For this review, take the finished solid that the model builds, in its own axes (mm). A direction names the side the tool comes from. Give positions to 0.01 mm unless a question says otherwise; leave off trailing zeros. Order: outer loops, then holes, each group sorted by start corner. A loop starts at its lowest first (then second) coordinate and runs counter-clockwise, first axis right, second up.
from build123d import *

# Parameters (mm, degrees)
F1_DEPTH = 25
F2_R     = 2
F4_DEPTH = 25


with BuildPart() as f1:
    # F0 (on Front) → F1 (new body)
    with BuildSketch(Plane.XZ):
        Polygon((3, 0), (0, 0), (-3, 0), (-3, -1), (-5, -3), (5, -3), (3, -1), align=None)
        Polygon((-3, 0), (0, 0), (3, 0), (3, 1), (-3, 1), align=None)
    extrude(amount=F1_DEPTH)

    # F2
    f2_edges = [f1.edges().sort_by_distance(p)[0] for p in [
        (-3, -25, 0),
        (-4, -25, -2),
        (4, -25, -2),
        (3, -25, 0),
        (-4, 0, -2),
        (3, 0, 0),
        (4, 0, -2),
        (-3, 0, 0),
    ]]
    fillet(f2_edges, radius=F2_R)

    # F3 (on face) → F4 (cut)
    with BuildSketch(Plane.XY.offset(1)):
        Polygon((-3, -12.972297), (-3, -12.5), (-3, -12.29), (-7.69, -12.29), (-7.69, -19.71), (-6.344625, -19.71), align=None)
        Polygon((-7.48, -12.5), (-3, -12.5), (-6.47483, -19.5), (-7.48, -19.5), align=None, mode=Mode.SUBTRACT)
        Polygon((-6.47483, -19.5), (-3, -12.5), (-7.48, -12.5), (-7.48, -19.5), align=None)
    extrude(amount=-F4_DEPTH, mode=Mode.SUBTRACT)


solid = f1.part
1) Tool access review of faces 4 (the face through (-2.43, -0.6, -0.12)), 5 (the face through (-3.5, -12.29, -2.4)), 6 (the face through (2.43, -24.4, -0.08)), 7 (the face through (2.43, -0.6, -0.08)), 8 (the face through (3, -12, 0)): name each direction out of +Z, -Z, +X, -X, +Y, -Y from which nothing blocks a thin tool from reaching the whole face with its end or side.
Answer sheet:
face 4: +Z, -X, +Y
face 5: +Z, -Z, -X
face 6: +Z, +X, -Y
face 7: +Z, +X, +Y
face 8: +Z, +X, +Y, -Y
2) We need section A-A on y = -15.75. Give the boundary of the cut face in (x, z).
Answer sheet:
outline: (-4.38, -3) - (5, -3) - (3, -1) - (3, 1) - (-3, 1) - (-3, -1) - (-4.38, -2.38) - close
3) To check wall thickness, follow line 1 (X direction, y = -21, z = -0.85); line 2 (Z direction, x = -4, y = -15.5); line 3 (X direction, y = -19.5, z = -2.5). State the ranges of each line that lie inside material, in increasing order.
Answer sheet:
line 1: x = -3 to 3
line 2: z = -3 to -2
line 3: x = -4.5 to 4.5
4) We need section C-C on y = -10.5. Give the boundary of the cut face in (x, z), then the cut area to 3 significant figures.
Answer sheet:
outline: (-5, -3) - (5, -3) - (3, -1) - (3, 1) - (-3, 1) - (-3, -1) - close
area: 28.0 mm2
5) We need section B-B on z = -0.6. Give the boundary of the cut face in (x, y), then the cut area to 3 significant figures.
Answer sheet:
outline: (-3, -23) arc R2 ccw to (-1, -25) - (1, -25) arc R2 ccw to (3, -23) - (3, -2) arc R2 ccw to (1, 0) - (-1, 0) arc R2 ccw to (-3, -2) - close
area: 147 mm2
6) Clearance check with flat-ended pins moving along their axes: pin 1 (2 mm diameter, centred on x = -4, z = -2.5, fed in from -Y); pin 2 (1 mm diameter, centred on y = -16.5, z = 0, fed in from +X); pin 3 (1 mm diameter, centred on y = -3, z = -1, fed in from +X). State where each tip first meets the part, or that it passes through.
Answer sheet:
pin 1: stops at y = -24.88
pin 2: stops at x = 3
pin 3: stops at x = 3.5
7) Draft analysis for pull direction Y (two halves, no side actions). For faces 1 (the face through (-2.43, -24.4, -0.12)), 2 (the face through (-3.32, -0.6, -2.13)), 3 (the face through (-3.57, -14.12, -2.43)), state which applies: +Y half, -Y half, draft (parallel to the pull), parting line (faces both ways), or undercut.
Answer sheet:
face 1: -Y half
face 2: +Y half
face 3: undercut
